from build123d import *

# Parameters (mm, degrees)
SKETCH1_W           = 73.9
SKETCH1_H           = 328
BOSS_EXTRUDE1_DEPTH = 5
SKETCH2_R           = 2.1
CUT_EXTRUDE1_DEPTH  = 10
CUT_EXTRUDE2_DEPTH  = 10
SKETCH5_R           = 2.1
CUT_EXTRUDE3_DEPTH  = 5
SKETCH6_R           = 2.1
SKETCH6_W           = 13
SKETCH6_H           = 10.5
CUT_EXTRUDE4_DEPTH  = 180
SKETCH7_R           = 2.1
CUT_EXTRUDE5_DEPTH  = 180
SKETCH8_W           = 40
SKETCH8_H           = 5
CUT_EXTRUDE6_DEPTH  = 5


with BuildPart() as part:
    # Sketch1 → Boss-Extrude1 (new body)
    with BuildSketch(Plane.XY):
        Rectangle(SKETCH1_W, SKETCH1_H)
    extrude(amount=BOSS_EXTRUDE1_DEPTH)

    # Sketch2 → Cut-Extrude1 (cut)
    with BuildSketch(Plane.XY.offset(5)):
        with Locations((-0.000417228, -81.5)):
            Circle(SKETCH2_R)
    extrude(amount=-CUT_EXTRUDE1_DEPTH, mode=Mode.SUBTRACT)

    # Sketch3 → Cut-Extrude2 (cut)
    with BuildSketch(Plane.XY.offset(5)):
        Polygon((-2.1, -164), (-2.1, -159), (-5, -159), (-5, -149), (5, -149), (5, -159), (2.1, -159), (2.1, -164), align=None)
        Polygon((2.1, 164), (2.1, 159), (5, 159), (5, 149), (-5, 149), (-5, 159), (-2.1, 159), (-2.1, 164), align=None)
    extrude(amount=-CUT_EXTRUDE2_DEPTH, mode=Mode.SUBTRACT)

    # Sketch5 → Cut-Extrude3 (cut)
    with BuildSketch(Plane.XY.offset(5)):
        with Locations((-0.000417228, -106.5)):
            Circle(SKETCH5_R)
    extrude(amount=-CUT_EXTRUDE3_DEPTH, mode=Mode.SUBTRACT)

    # Sketch6 → Cut-Extrude4 (cut)
    with BuildSketch(Plane.XY.offset(5)):
        with Locations((-26.856574817, 38)):
            Circle(SKETCH6_R)
        with Locations((26.85574036, 38)):
            Circle(SKETCH6_R)
        with Locations((26.85574036, -72)):
            Circle(SKETCH6_R)
        with Locations((-26.856574817, -72)):
            Circle(SKETCH6_R)
        with Locations((0.059582772, 38)):
            Rectangle(SKETCH6_W, SKETCH6_H)
        with Locations((0.059582772, -72)):
            Rectangle(SKETCH6_W, SKETCH6_H)
    extrude(amount=-CUT_EXTRUDE4_DEPTH, mode=Mode.SUBTRACT)

    # Sketch7 → Cut-Extrude5 (cut)
    with BuildSketch(Plane(origin=(0, 0, 0), x_dir=(-1, 0, 0), z_dir=(0, 0, -1))):
        with Locations((11.250417228, 38)):
            Circle(SKETCH7_R)
        with Locations((-11.249582772, 38)):
            Circle(SKETCH7_R)
        with Locations((-11.249582772, -72)):
            Circle(SKETCH7_R)
        with Locations((11.250417228, -72)):
            Circle(SKETCH7_R)
    extrude(amount=-CUT_EXTRUDE5_DEPTH, mode=Mode.SUBTRACT)

    # Sketch8 → Cut-Extrude6 (cut)
    with BuildSketch(Plane.XY.offset(5)):
        with Locations((-0.000417229, -26.5)):
            Rectangle(SKETCH8_W, SKETCH8_H)
    extrude(amount=-CUT_EXTRUDE6_DEPTH, mode=Mode.SUBTRACT)


solid = part.part
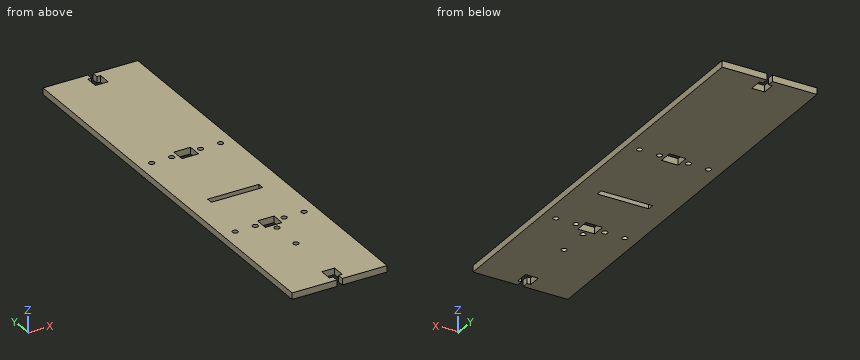
Model file for the job. Use its own axes, mm. Give positions to 0.01 mm unless a question says otherwise; leave off trailing zeros. One line per item, written item: value.
Item 1: Wall check: line 1 (Y direction, x = 11.5, z = 3.3); line 2 (Y direction, x = -27, z = 0.5); line 3 (Y direction, x = 3, z = 0.8). Give the ranges that are in metal, low to high.
Response values:
line 1: -164 to -74.09, -69.91 to -29, -24 to 35.91, 40.09 to 164
line 2: -164 to -74.1, -69.9 to 35.9, 40.1 to 164
line 3: -164 to -159, -149 to -77.25, -66.75 to -29, -24 to 32.75, 43.25 to 149, 159 to 164
Item 2: Pin check, flat tips, straight feed: pin 1 Ø1.5 at (x, y) = (1.5, -81) entering from -Z; pin 2 Ø1.5 at (x, z) = (-0.5, 1.5) entering from -Y; pin 3 Ø2.5 at (x, y) = (0, -106.5) entering from -Z. Stop position of each tip, or through.
Response values:
pin 1: z = 0
pin 2: y = -149
pin 3: through
Item 3: Slice it at A-A (z = 2.25). Give the number of separate pieces and of enclosed holes in the cut face, then the cut area to 3 significant figures.
Response values:
separate pieces: 1
enclosed holes: 13
area: 23,400 mm2
